Could you check a few things on this model? Use its own coordinates, in mm. Give positions to 0.01 mm unless a question says otherwise; leave off trailing zeros. Loops run counter-clockwise (first coordinate to the right, second up) from the corner with the lowest first, then second, coordinate; pieces in that order, holes last. Notation, with made-up numbers: (43, -13) -> (68, -13) arc R18 cw to (68, 15) -> close; hole circle Ø6 at (89.5, -25). An arc over 180 degrees is marked (long way). Put each result on its own line as item: value.
```python
from build123d import *

# Parameters (mm, degrees)
SKETCH1_R           = 1.5
BOSS_EXTRUDE1_DEPTH = 3
SKETCH2_W           = 26.5
SKETCH2_H           = 13.12704922
BOSS_EXTRUDE2_DEPTH = 3
SKETCH3_R           = 1.5
CUT_EXTRUDE1_DEPTH  = 10
SKETCH4_R           = 1.5
CUT_EXTRUDE2_DEPTH  = 10


with BuildPart() as part:
    # Sketch1 → Boss-Extrude1 (new body)
    with BuildSketch(Plane(origin=(0, 0, 0), x_dir=(1, 0, 0), z_dir=(0, 1, 0))):
        Polygon((-5, -5), (41.5, -5), (41.5, 64.6), (31.5, 64.6), (-5, 56.73), align=None)
        Polygon((31.5, 54.48), (31.5, 5.234024539), (5, 5.234024539), (5, 56.73), align=None, mode=Mode.SUBTRACT)
        Circle(SKETCH1_R, mode=Mode.SUBTRACT)
        with Locations((0, 51.73)):
            Circle(SKETCH1_R, mode=Mode.SUBTRACT)
        with Locations((36.5, 59.6)):
            Circle(SKETCH1_R, mode=Mode.SUBTRACT)
        with Locations((36.5, 11.18)):
            Circle(SKETCH1_R, mode=Mode.SUBTRACT)
        with Locations((36.5, 49.6)):
            Circle(SKETCH1_R, mode=Mode.SUBTRACT)
    extrude(amount=BOSS_EXTRUDE1_DEPTH)

    # Sketch2 → Boss-Extrude2 (add)
    with BuildSketch(Plane(origin=(0, 3, 0), x_dir=(1, 0, 0), z_dir=(0, 1, 0))):
        with Locations((18.25, 37.545536879)):
            Rectangle(SKETCH2_W, SKETCH2_H)
        Polygon((5, 56.73), (5, 49.867078553), (31.5, 54.48), align=None)
    extrude(amount=-BOSS_EXTRUDE2_DEPTH)

    # Sketch3 → Cut-Extrude1 (cut)
    with BuildSketch(Plane(origin=(0, 3, 0), x_dir=(1, 0, 0), z_dir=(0, 1, 0))):
        with Locations((10, 0)):
            Circle(SKETCH3_R)
    extrude(amount=-CUT_EXTRUDE1_DEPTH, mode=Mode.SUBTRACT)

    # Sketch4 → Cut-Extrude2 (cut)
    with BuildSketch(Plane(origin=(0, 3, 0), x_dir=(1, 0, 0), z_dir=(0, 1, 0))):
        with Locations((0, 8)):
            Circle(SKETCH4_R)
    extrude(amount=-CUT_EXTRUDE2_DEPTH, mode=Mode.SUBTRACT)


solid = part.part
```
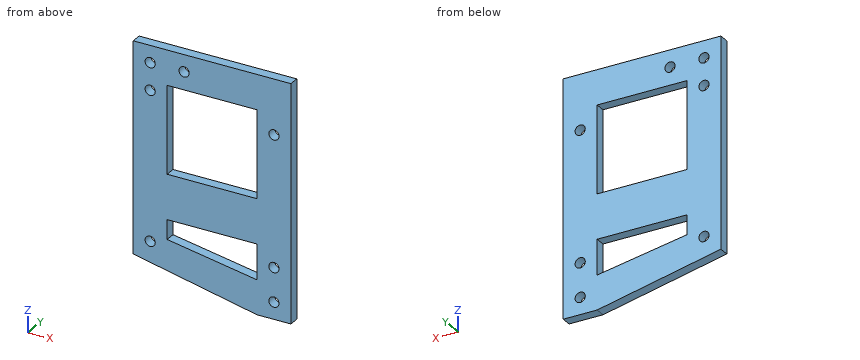
1. If we section it at A-A (x = 36.5): List the corners of the cut face in (y, z) for me, then the cut area to 3 significant figures.
Recorded:
outline: (0, -64.6) -> (3, -64.6) -> (3, -61.1) -> (0, -61.1) -> close; (0, -58.1) -> (3, -58.1) -> (3, -51.1) -> (0, -51.1) -> close; (0, -48.1) -> (3, -48.1) -> (3, -12.68) -> (0, -12.68) -> close; (0, -9.68) -> (3, -9.68) -> (3, 5) -> (0, 5) -> close
area: 182 mm^2
2. I need wall thicknesses on line 1 (Z direction, x = 25, y = 1.75); line 2 (Z direction, x = 0, y = 0.9); line 3 (Z direction, x = 36.5, y = 1.35). Which ranges of each line are inside material? Lowest first, please.
Recorded:
line 1: z = -63.2 to -53.35, -44.11 to -30.98, -5.23 to 5
line 2: z = -57.81 to -53.23, -50.23 to -9.5, -6.5 to -1.5, 1.5 to 5
line 3: z = -64.6 to -61.1, -58.1 to -51.1, -48.1 to -12.68, -9.68 to 5
3. If we section it at B-B (z = -18.5): List the corners of the cut face in (x, y) for me, then the cut area to 3 significant figures.
Recorded:
outline: (-5, 0) -> (5, 0) -> (5, 3) -> (-5, 3) -> close; (31.5, 0) -> (41.5, 0) -> (41.5, 3) -> (31.5, 3) -> close
area: 60.0 mm^2
4. If we section it at D-D (y = 2.3): Count the separate pieces of the cut face and the enclosed holes in it, then the cut area to 3 significant figures.
Recorded:
separate pieces: 1
enclosed holes: 9
area: 2,150 mm^2
5. If we section it at C-C (z = -8): List the corners of the cut face in (x, y) for me.
Recorded:
outline: (-5, 0) -> (-1.5, 0) -> (-1.5, 3) -> (-5, 3) -> close; (1.5, 0) -> (5, 0) -> (5, 3) -> (1.5, 3) -> close; (31.5, 0) -> (41.5, 0) -> (41.5, 3) -> (31.5, 3) -> close
6. I'm going to push flat-ended pins straight in: pin 1 (1.5 mm diameter, centred on x = 23.5, y = 1.5, fed in from -Z); pin 2 (1.5 mm diameter, centred on x = 5, y = 0.5, fed in from -Z). Where does each tip first touch, or does it pass through?
Recorded:
pin 1: stops at z = -63.04
pin 2: stops at z = -59.05
